Answer from the drawing. Dimensions are ordinates in mm from the lowest x, y and z of the part. Give positions to 0.01 mm unless a question says otherwise; leave off trailing zeros. Write each loop counter-clockwise with the first axis right and the second up, starting at its lowest first coordinate (ties: lowest second). Pieces come first, ordered by that corner, then holes. Notation, with made-up numbers: (-29.75, 28.25) -> (-15.75, 28.25) arc R23 cw to (-15.75, 65.25) -> close; hole circle Ø10 at (-39.75, 75.25). An arc over 180 degrees is marked (long way). Put each result on its own line as item: value. Start each with the question number.
1) Flat-ended cylindrical pins translate along their axes: pin 1 Ø0.8 at (x, z) = (1.5, 22.5) entering from -Y; pin 2 Ø2 at (x, z) = (1, 20) entering from +Y; pin 3 Ø1.2 at (x, y) = (1, 25.5) entering from +Z. Find the tip coordinate at first contact, or state that the pin passes through.
2) For a pull along Y with two mould halves and no side action, classify the marked faces 1 and 2 as released by +Y, released by -Y, zero draft, split by the parting line, or undercut.
3) A cutting plane is placed at D-D (z = 46). Write down the section's boundary in (x, y), then the cut area to 3 significant figures.
4) A cutting plane is placed at A-A (x = 1.5). Write down the section's boundary in (y, z).
5) A cutting plane is placed at B-B (y = 29). Write down the section's boundary in (x, z).
6) Find the intervals of material crossed by line 1 along Z through (x, y) = (2.2, 29); line 2 along X through (y, z) = (32.5, 15.5), in increasing order. Write a range as from..to.
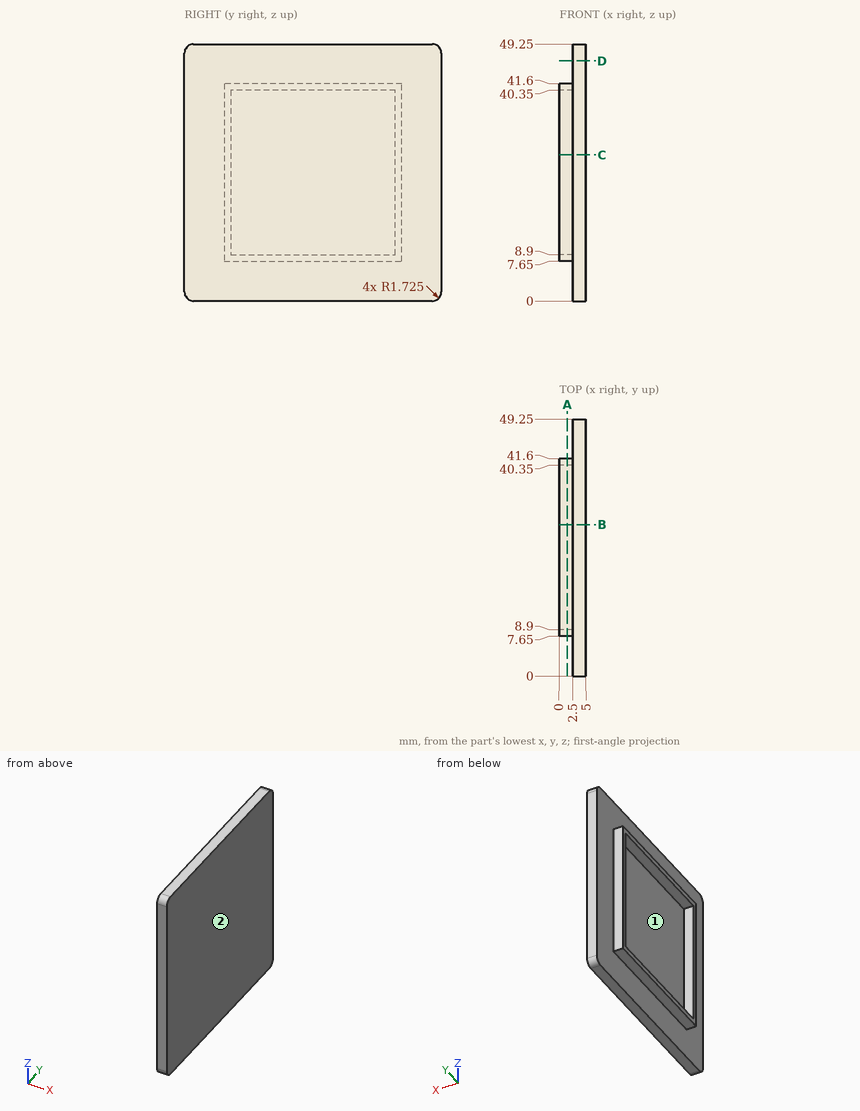
Reply:
1. pin 1: stops at y = 7.65
1. pin 2: stops at y = 41.6
1. pin 3: stops at z = 41.6
2. face 1: undercut
2. face 2: zero draft
3. outline: (2.5, 0) -> (5, 0) -> (5, 49.25) -> (2.5, 49.25) -> close
3. area: 123 mm2
4. outline: (7.65, 7.65) -> (41.6, 7.65) -> (41.6, 41.6) -> (7.65, 41.6) -> close; hole (8.9, 8.9) -> (40.35, 8.9) -> (40.35, 40.35) -> (8.9, 40.35) -> close
5. outline: (0, 7.65) -> (2.5, 7.65) -> (2.5, 0) -> (5, 0) -> (5, 49.25) -> (2.5, 49.25) -> (2.5, 41.6) -> (0, 41.6) -> (0, 40.35) -> (2.5, 40.35) -> (2.5, 8.9) -> (0, 8.9) -> close
6. line 1: z = 7.65..8.9, 40.35..41.6
6. line 2: x = 2.5..5
